```python
from build123d import *

# Parameters (mm, degrees)
SKETCH1_W           = 15.5
SKETCH1_H           = 7.75
BOSS_EXTRUDE1_DEPTH = 6.4


with BuildPart() as part:
    # Sketch1 → Boss-Extrude1 (new body)
    with BuildSketch(Plane(origin=(0, 0, 0), x_dir=(1, 0, 0), z_dir=(0, 1, 0))):
        Polygon((136.176, 177.3), (166.73, 177.3), (174.23, 169.8), (174.23, -112.7), (166.73, -120.2), (-29.725, -120.2), (-29.725, 25.249320413), (-24.025, 25.249320413), (-24.025, 24.000679587), (-22.225, 24.000679587), (-22.225, 25.249320413), (-18.825, 25.249320413), (-18.825, 28.900679587), (-22.225, 28.900679587), (-22.225, 30.150679587), (-24.025, 30.150679587), (-24.025, 28.900679587), (-29.725, 28.900679587), (-29.725, 147.3), (0.275, 177.3), (29.906, 177.3), (29.906, 182.7), (22.906, 184.689990555), (22.941578202, 189.687449255), (35.946, 189.687449255), (37.946, 187.687449255), (37.946, 177.3), (128.136, 177.3), (128.136, 182.7), (121.136, 184.689990555), (121.171578202, 189.687449255), (134.176, 189.687449255), (136.176, 187.687449255), align=None)
        with Locations((123.48, -35.75)):
            Rectangle(SKETCH1_W, SKETCH1_H, mode=Mode.SUBTRACT)
        with Locations((25.25, -35.75)):
            Rectangle(SKETCH1_W, SKETCH1_H, mode=Mode.SUBTRACT)
        Polygon((164.957922061, 82.8), (164.957922061, 80.8), (169.23, 76.527922061), (169.23, 69.072077939), (164.957922061, 64.8), (164.957922061, 62.8), (169.23, 58.527922061), (169.23, 51.072077939), (163.957922061, 45.8), (151.23, 45.8), (151.23, 99.8), (163.957922061, 99.8), (169.23, 94.527922061), (169.23, 87.072077939), align=None, mode=Mode.SUBTRACT)
    extrude(amount=BOSS_EXTRUDE1_DEPTH)


solid = part.part
```
Input: part model. Units: mm. Frame: model coordinates. A direction names the side the tool comes from. Give positions to 0.01 mm unless a question says otherwise; leave off trailing zeros. Write each loop counter-clockwise with the first axis right and the second up, starting at its lowest first coordinate (ties: lowest second). Pieces come first, ordered by that corner, then holes. Notation, with made-up numbers: (-9.75, -31.5) - (30.25, -31.5) arc R18 ccw to (30.25, -22.5) - close; hole circle Ø1 at (49, -16). An arc over 180 degrees is marked (long way). Write item = value, one per line. Start each with the question number.
1) Cut plane B-B (x = 98). Return loops of the section in (y, z).
2) Material intervals for L1, parallel to X at y = 3, z = -53.5 (3 decimals); L2, parallel to Z at x = 26, y = 1.25 (3 decimals); L3, parallel to Z at x = 119.5, y = 3.5 (3 decimals), sorted ascending. Write a range as [from, to].
3) Pin query (flat end, axial travel): pin 1 (1 mm diameter, centred on x = 107.5, y = 2.5, fed in from -Z); pin 2 (2.5 mm diameter, centred on y = 4, z = -179, fed in from -X). Return the tip coordinate at first contact, or that it passes through.
4) Cut plane A-A (y = 4.5). Give the number of separate pieces and of enclosed holes in the cut face, and give its area (3 significant figures).
5) Cut plane C-C (x = -3.5). Return loops of the section in (y, z) (3 decimals), and give its area (3 significant figures).
6) Draft query along Z for faces 1 (the face through (128, 3, -189.687)), 2 (the face through (15, 3, -177.3)), 3 (the face through (74, 6.4, -37)), 4 (the face through (25, 3, 39.625)). Return one class per face: pulls with the +Z half, pulls with the -Z half, needs draft (parallel to the pull), parting line crosses it, or undercut.
7) Reachability of faces 5 (the face through (169.23, 3, -91)), 6 (the face through (26.46, 3.16, -183.68)), 7 (the face through (151, 3, -177.3)) from +Z, -Z, +X, -X, +Y, -Y: full face, straight path, thin tool, end or side. Return the list, or none.
Answers follow:
q1.outline = (0, -177.3) - (6.4, -177.3) - (6.4, 120.2) - (0, 120.2) - close
q2.L1 = [-29.725, 151.23], [169.23, 174.23]
q2.L2 = [-189.687, -183.81], [-177.3, 31.875], [39.625, 120.2]
q2.L3 = [-177.3, 31.875], [39.625, 120.2]
q3.pin_1 = -177.3
q3.pin_2 = 29.91
q4.separate_pieces = 1
q4.enclosed_holes = 3
q4.area = 59,300 mm^2
q5.outline = (0, -173.525) - (6.4, -173.525) - (6.4, 120.2) - (0, 120.2) - close
q5.area = 1,880 mm^2
q6.face_1 = pulls with the -Z half
q6.face_2 = undercut
q6.face_3 = needs draft
q6.face_4 = undercut
q7.face_5 = +Y, -Y
q7.face_6 = -X, +Y, -Y
q7.face_7 = -Z, +X, +Y, -Y
